Design review of the part built by this model. Coordinates are the model's own, in mm. Face numbers are marked on the shaded views. A direction names the side the tool comes from. Round coordinates to 2 decimals unless told otherwise and drop trailing zeros. Loops run counter-clockwise (first coordinate to the right, second up) from the corner with the lowest first, then second, coordinate; pieces in that order, holes last. Notation, with made-up numbers: (37, 13.25) - (61, 13.25) arc R24 cw to (61, 31.25) - close; hole circle Ø8 at (-4, -5.5). An arc over 180 degrees is marked (long way). Return JSON: item names as keys, results as strings. Group by question number.
(1) We need section D-D, the plane x = 6. Write out the cut boundary in (y, z).
(2) Wall thickness on L1, parallel to X at y = 4.3, z = 0; L2, parallel to X at y = 1.1, z = 6.25; L3, parallel to X at y = 1.55, z = 0.75: over which ranges is each line inside the solid? List them lowest first. Write a range as [from, to].
(3) We need section B-B, the plane y = 2. Write out the cut boundary in (x, z), and give its area (3 significant figures).
(4) We need section A-A, the plane x = 0. Write out the cut boundary in (y, z).
(5) Clearance check with flat-ended pins moving along their axes: pin 1 (0.5 mm diameter, centred on x = 0.5, y = 1.5, fed in from -Z); pin 2 (9.5 mm diameter, centred on x = 0, z = 0, fed in from +Y); pin 3 (1 mm diameter, centred on x = 5, y = 1.5, fed in from +Z). State where each tip first meets the part, or that it passes through.
(6) We need section C-C, the plane z = 6. Write out the cut boundary in (x, y), and give its area (3 significant figures).
(7) For the marked faces 1, 2 and 3, list the 3-axis set-ups (+Z, -Z, +X, -X, +Y, -Y) from which the entire face can be reached by the end or side of a thin tool; tool diameter is ignored.
(8) The part is to be moulded in two halves that separate along Z. For the marked faces 4, 5 and 6, say which applies: pulls with the +Z half, pulls with the -Z half, needs draft (parallel to the pull), parting line crosses it, or undercut.
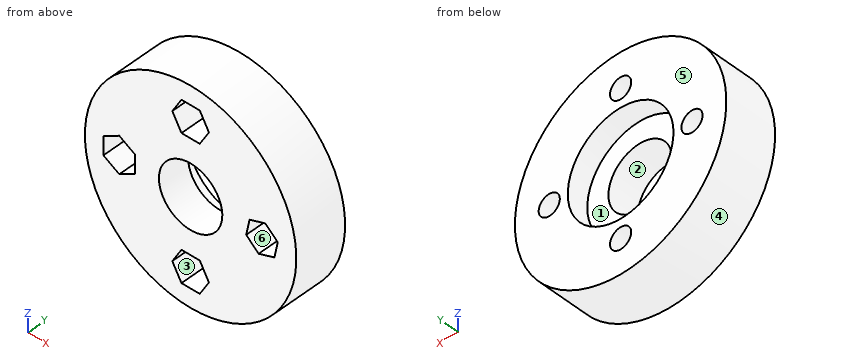
from build123d import *

# Parameters (mm, degrees)
SKETCH1_R           = 5
SKETCH1_R_2         = 3
BOSS_EXTRUDE1_DEPTH = 3
SKETCH1_3_R         = 10
SKETCH1_3_R_2       = 5
BOSS_EXTRUDE2_DEPTH = 5
BOSS_EXTRUDE3_START = 3
SKETCH1_4_R         = 1
BOSS_EXTRUDE3_DEPTH = 2


with BuildPart() as part:
    # Sketch1 → Boss-Extrude1 (new body)
    with BuildSketch(Plane(origin=(0, 0, 0), x_dir=(1, 0, 0), z_dir=(0, 1, 0))):
        with Locations(Location((0, 0, 0), (0, 0, 270))):
            Circle(SKETCH1_R)
        with Locations(Location((0, 0, 0), (0, 0, 270))):
            Circle(SKETCH1_R_2, mode=Mode.SUBTRACT)
    extrude(amount=BOSS_EXTRUDE1_DEPTH)

    # Sketch1_3 → Boss-Extrude2 (add)
    with BuildSketch(Plane(origin=(0, 0, 0), x_dir=(1, 0, 0), z_dir=(0, 1, 0))):
        with Locations(Location((0, 0, 0), (0, 0, 270))):
            Circle(SKETCH1_3_R)
        with Locations(Location((0, 0, 0), (0, 0, 270))):
            Circle(SKETCH1_3_R_2, mode=Mode.SUBTRACT)
        Polygon((-8.25, -0.866025404), (-6.75, -1.732050808), (-5.25, -0.866025404), (-5.25, 0.866025404), (-6.75, 1.732050808), (-8.25, 0.866025404), align=None, mode=Mode.SUBTRACT)
        Polygon((0.866025404, 5.25), (1.732050808, 6.75), (0.866025404, 8.25), (-0.866025404, 8.25), (-1.732050808, 6.75), (-0.866025404, 5.25), align=None, mode=Mode.SUBTRACT)
        Polygon((7.067372744, -1.54054846), (8.242840474, -0.495421371), (7.92546773, 1.045127089), (6.432627256, 1.54054846), (5.257159526, 0.495421371), (5.57453227, -1.045127089), align=None, mode=Mode.SUBTRACT)
        Polygon((0.866025404, -8.25), (1.732050808, -6.75), (0.866025404, -5.25), (-0.866025404, -5.25), (-1.732050808, -6.75), (-0.866025404, -8.25), align=None, mode=Mode.SUBTRACT)
    extrude(amount=BOSS_EXTRUDE2_DEPTH)

    # Sketch1_4 → Boss-Extrude3 (add)
    # profile 1 of 4: a face of its own
    with BuildSketch(Plane(origin=(0, 0, 0), x_dir=(1, 0, 0), z_dir=(0, 1, 0)).offset(BOSS_EXTRUDE3_START)):
        Polygon((-0.866025404, -8.25), (0.866025404, -8.25), (1.732050808, -6.75), (0.866025404, -5.25), (-0.866025404, -5.25), (-1.732050808, -6.75), align=None)
        with Locations(Location((0, -6.75, 0), (0, 0, 270))):
            Circle(SKETCH1_4_R, mode=Mode.SUBTRACT)
    # profile 2 of 4: a face of its own
    with BuildSketch(Plane(origin=(0, 0, 0), x_dir=(1, 0, 0), z_dir=(0, 1, 0)).offset(BOSS_EXTRUDE3_START)):
        Polygon((5.57453227, -1.045127089), (7.067372744, -1.54054846), (8.242840474, -0.495421371), (7.92546773, 1.045127089), (6.432627256, 1.54054846), (5.257159526, 0.495421371), align=None)
        with Locations(Location((6.75, 0, 0), (0, 0, 270))):
            Circle(SKETCH1_4_R, mode=Mode.SUBTRACT)
    # profile 3 of 4: a face of its own
    with BuildSketch(Plane(origin=(0, 0, 0), x_dir=(1, 0, 0), z_dir=(0, 1, 0)).offset(BOSS_EXTRUDE3_START)):
        Polygon((-0.866025404, 5.25), (0.866025404, 5.25), (1.732050808, 6.75), (0.866025404, 8.25), (-0.866025404, 8.25), (-1.732050808, 6.75), align=None)
        with Locations(Location((0, 6.75, 0), (0, 0, 270))):
            Circle(SKETCH1_4_R, mode=Mode.SUBTRACT)
    # profile 4 of 4: a face of its own
    with BuildSketch(Plane(origin=(0, 0, 0), x_dir=(1, 0, 0), z_dir=(0, 1, 0)).offset(BOSS_EXTRUDE3_START)):
        Polygon((-8.25, 0.866025404), (-8.25, -0.866025404), (-6.75, -1.732050808), (-5.25, -0.866025404), (-5.25, 0.866025404), (-6.75, 1.732050808), align=None)
        with Locations(Location((-6.75, 0, 0), (0, 0, 270))):
            Circle(SKETCH1_4_R, mode=Mode.SUBTRACT)
    extrude(amount=BOSS_EXTRUDE3_DEPTH)


solid = part.part
Solutions:
{
 "1": {"outline": "(0, -8) - (5, -8) - (5, -0.66) - (3, -0.66) - (3, -1.16) - (0, -1.16) - close; (0, 1.19) - (3, 1.19) - (3, 0.66) - (5, 0.66) - (5, 8) - (0, 8) - close"},
 "2": {"L1": "[-10, -7.75], [-5.75, -5], [5, 5.75], [7.75, 10]", "L2": "[-7.81, -1.44], [1.44, 7.81]", "L3": "[-9.97, -8.25], [-5.25, -2.9], [2.9, 5.51], [7.96, 9.97]"},
 "3": {"outline": "circle Ø20 at (0, 0); hole (-8.25, -0.87) - (-6.75, -1.73) - (-5.25, -0.87) - (-5.25, 0.87) - (-6.75, 1.73) - (-8.25, 0.87) - close; hole circle Ø6 at (0, 0); hole (-1.73, -6.75) - (-0.87, -8.25) - (0.87, -8.25) - (1.73, -6.75) - (0.87, -5.25) - (-0.87, -5.25) - close; hole (-1.73, 6.75) - (-0.87, 5.25) - (0.87, 5.25) - (1.73, 6.75) - (0.87, 8.25) - (-0.87, 8.25) - close; hole (5.26, -0.5) - (6.43, -1.54) - (7.93, -1.05) - (8.24, 0.5) - (7.07, 1.54) - (5.57, 1.05) - close", "area": "256 mm^2"},
 "4": {"outline": "(0, -10) - (5, -10) - (5, -7.75) - (3, -7.75) - (3, -8.25) - (0, -8.25) - close; (0, -5.25) - (3, -5.25) - (3, -5.75) - (5, -5.75) - (5, -5) - (3, -5) - (3, -3) - (0, -3) - close; (0, 3) - (3, 3) - (3, 5) - (5, 5) - (5, 5.75) - (3, 5.75) - (3, 5.25) - (0, 5.25) - close; (0, 8.25) - (3, 8.25) - (3, 7.75) - (5, 7.75) - (5, 10) - (0, 10) - close"},
 "5": {"pin 1": "z = -10", "pin 2": "y = 3", "pin 3": "z = 8.93"},
 "6": {"outline": "(-8, 0) - (-1.3, 0) - (-1.3, 3) - (-0.66, 3) - (-0.66, 5) - (-8, 5) - close; (0.66, 3) - (1.3, 3) - (1.3, 0) - (8, 0) - (8, 5) - (0.66, 5) - close", "area": "69.6 mm^2"},
 "7": {"face 1": "+Y", "face 2": "+Y, -Y", "face 3": "-Y"},
 "8": {"face 4": "parting line crosses it", "face 5": "needs draft", "face 6": "undercut"}
}
